The model under review builds one solid part; all positions refer to its coordinate system, in mm. Face numbers are marked on the shaded views. Coordinates: 2 decimals unless noted, no trailing zeros. Order: outer loops, then holes, each group sorted by start corner. A loop starts at its lowest first (then second) coordinate and runs counter-clockwise, first axis right, second up. Notation, with made-up numbers: (-37, -21.75) -> (-16, -21.75) arc R27 ccw to (-16, 15.25) -> close; hole circle Ø5 at (-23.5, 66). An arc over 180 degrees is marked (long way). Use one line per item in the form item = value. Start each with the question number.
(1) Mouldability with a two-part tool opening along Y and no side actions: class the marked faces 1 and 2 as +Y half, -Y half, draft (parallel to the pull), parting line (faces both ways), or undercut.
(2) Wall thickness on line 1 along Z through (x, y) = (-11.5, 4) (3 decimals); line 2 along X through (y, z) = (3.25, 2): over which ranges is each line inside the solid? List them lowest first.
(3) Take a section at A-A (x = 44). State the section outline as (y, z) points (3 decimals), then the cut area to 3 significant figures.
(4) Insertion check: pin 1 Ø3 at (y, z) = (3, 34.5) entering from -X; pin 2 Ø1.7 at (x, y) = (-48.5, 4) entering from +Z; pin 3 Ø2.5 at (x, y) = (-48.5, 4.5) entering from +Z. Each pin has a flat end and moves straight along its axis. Give the tip position at first contact, or say it passes through.
(5) Take a section at B-B (z = 14.5). State the section outline as (x, y) points, then the cut area to 3 significant figures.
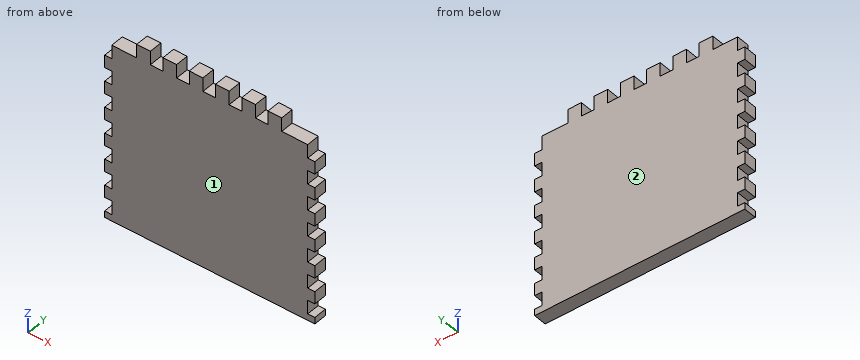
```python
from build123d import *

# Parameters (mm, degrees)
SKETCH1_W               = 101.6
SKETCH1_H               = 107.95
BOSS_EXTRUDE1_DEPTH     = 6.35
CUT_EXTRUDE1_DEPTH      = 75.392628163
CUT_EXTRUDE1_DEPTH_BACK = 75.392628163
SKETCH2_W               = 3.429
SKETCH2_H               = 6.604


with BuildPart() as part:
    # Sketch1 → Boss-Extrude1 (new body)
    with BuildSketch(Plane(origin=(0, 0, 0), x_dir=(1, 0, 0), z_dir=(0, 1, 0))):
        Rectangle(SKETCH1_W, SKETCH1_H)
    extrude(amount=BOSS_EXTRUDE1_DEPTH)

    # Sketch2 → Cut-Extrude1 (cut, two sides: drawn at the far end of the back side and taken through both)
    with BuildSketch(Plane(origin=(0, 6.35, 0), x_dir=(1, 0, 0), z_dir=(0, 1, 0)).offset(-CUT_EXTRUDE1_DEPTH_BACK)):
        Polygon((22.098, -31.877), (28.194, -31.877), (28.194, -38.481), (34.798, -38.481), (34.798, -31.877), (47.371, -31.877), (47.371, -25.273), (50.8, -25.273), (50.8, -31.877), (50.8, -53.975), (-50.8, -53.975), (-50.8, -31.877), (-50.8, -25.273), (-47.371, -25.273), (-47.371, -31.877), (-35.306, -31.877), (-35.306, -38.481), (-28.702, -38.481), (-28.702, -31.877), (-22.606, -31.877), (-22.606, -38.481), (-16.002, -38.481), (-16.002, -31.877), (-9.906, -31.877), (-9.906, -38.481), (-3.302, -38.481), (-3.302, -31.877), (2.794, -31.877), (2.794, -38.481), (9.398, -38.481), (9.398, -31.877), (15.494, -31.877), (15.494, -38.481), (22.098, -38.481), align=None)
        with Locations((-49.0855, 47.498)):
            Rectangle(SKETCH2_W, SKETCH2_H)
        with Locations((-49.0855, 34.925)):
            Rectangle(SKETCH2_W, SKETCH2_H)
        with Locations((-49.0855, 22.225)):
            Rectangle(SKETCH2_W, SKETCH2_H)
        with Locations((-49.0855, 9.525)):
            Rectangle(SKETCH2_W, SKETCH2_H)
        with Locations((-49.0855, -3.175)):
            Rectangle(SKETCH2_W, SKETCH2_H)
        with Locations((-49.0855, -15.875)):
            Rectangle(SKETCH2_W, SKETCH2_H)
        with Locations((49.0855, -15.875)):
            Rectangle(SKETCH2_W, SKETCH2_H)
        with Locations((49.0855, -3.175)):
            Rectangle(SKETCH2_W, SKETCH2_H)
        with Locations((49.0855, 9.525)):
            Rectangle(SKETCH2_W, SKETCH2_H)
        with Locations((49.0855, 22.225)):
            Rectangle(SKETCH2_W, SKETCH2_H)
        with Locations((49.0855, 34.925)):
            Rectangle(SKETCH2_W, SKETCH2_H)
        with Locations((49.0855, 47.498)):
            Rectangle(SKETCH2_W, SKETCH2_H)
    extrude(amount=CUT_EXTRUDE1_DEPTH + CUT_EXTRUDE1_DEPTH_BACK, mode=Mode.SUBTRACT)


solid = part.part
```
Findings:
q1.face_1 = -Y half
q1.face_2 = +Y half
q2.line_1 = -53.975 to 31.877
q2.line_2 = -47.37 to 47.37
q3.outline = (0, -53.975) -> (6.35, -53.975) -> (6.35, 31.877) -> (0, 31.877) -> close
q3.area = 545 mm²
q4.pin_1 = -35.31
q4.pin_2 = 25.27
q4.pin_3 = 31.88
q5.outline = (-47.37, 0) -> (47.37, 0) -> (47.37, 6.35) -> (-47.37, 6.35) -> close
q5.area = 602 mm²
